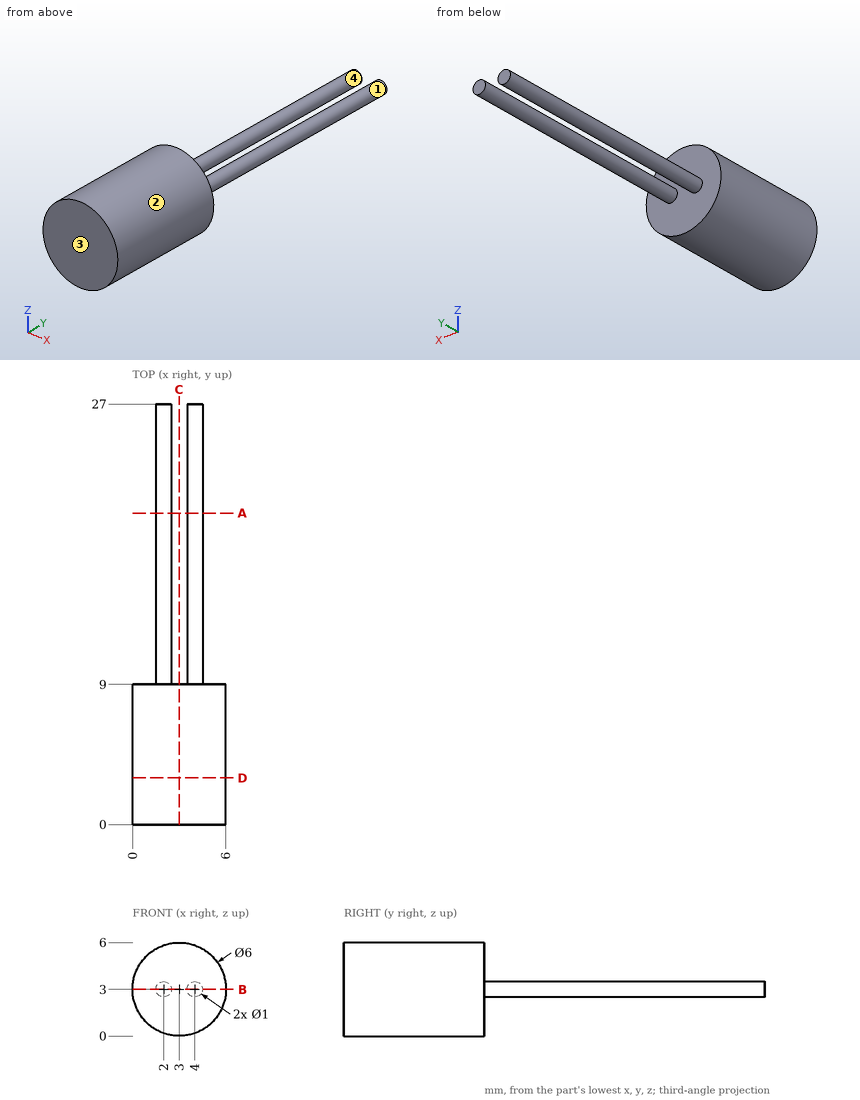
The figure shows three views and two pictorial views of one solid part (mm, origin at its lowest corner). Answer the questions. Coordinates: 2 decimals unless noted, no trailing zeros. Loops run counter-clockwise (first coordinate to the right, second up) from the corner with the lowest first, then second, coordinate; pieces in that order, holes last. Notation, with made-up numbers: (43, -22.75) -> (75, -22.75) arc R18 ccw to (75, -12.75) -> close; hole circle Ø8 at (9.5, 48). An arc over 180 degrees is marked (long way). Use one line per item in the form item = value. Start each with the question number.
Item 1: The mould has two halves that part along X. Classify the marked faces 1, 2, 3 and 4: released by +X, released by -X, zero draft, split by the parting line, or undercut.
Item 2: Consider L1, parallel to Y at x = 1, z = 1.6; L2, parallel to X at y = 7, z = 2.9; L3, parallel to Z at x = 4.15, y = 7.75. Determine where each line is inside the solid, lowest interval first. Write a range as [from, to].
Item 3: The part is cut by section C-C on x = 3. Determine the outline of the cut face in (y, z).
Item 4: The part is cut by section A-A on y = 20. Determine the outline of the cut face in (x, z).
Item 5: Flat-ended cylindrical pins translate along their axes: pin 1 Ø1 at (x, z) = (1.5, 3.5) entering from +Y; pin 2 Ø3 at (y, z) = (16.5, 3) entering from +X. Find the tip coordinate at first contact, or state that the pin passes through.
Item 6: The part is cut by section D-D on y = 3. Determine the outline of the cut face in (x, z).
Item 7: The part is cut by section B-B on z = 3. Determine the outline of the cut face in (x, y).
Answer key:
q1.face_1 = undercut
q1.face_2 = split by the parting line
q1.face_3 = zero draft
q1.face_4 = undercut
q2.L1 = [0, 9]
q2.L2 = [0, 6]
q2.L3 = [0.23, 5.77]
q3.outline = (0, 0) -> (9, 0) -> (9, 6) -> (0, 6) -> close
q4.outline = circle Ø1 at (2, 3); circle Ø1 at (4, 3)
q5.pin_1 = 27
q5.pin_2 = 4.5
q6.outline = circle Ø6 at (3, 3)
q7.outline = (0, 0) -> (6, 0) -> (6, 9) -> (4.5, 9) -> (4.5, 27) -> (3.5, 27) -> (3.5, 9) -> (2.5, 9) -> (2.5, 27) -> (1.5, 27) -> (1.5, 9) -> (0, 9) -> close
